```python
from build123d import *

# Parameters (mm, degrees)
SKETCH004_W     = 20
SKETCH004_H     = 8
PAD003_DEPTH    = 6
POCKET001_DEPTH = 5
SKETCH006_R     = 1.6
POCKET002_DEPTH = 11
FILLET004_R     = 3


with BuildPart() as part:
    # Sketch004 (on XY_Plane001 of Origin002) → Pad003 (new body)
    with BuildSketch(Plane.XY):
        Rectangle(SKETCH004_W, SKETCH004_H)
    extrude(amount=PAD003_DEPTH)

    # Sketch005 (on XZ_Plane001 of Origin002) → Pocket001 (cut, symmetric)
    with BuildSketch(Plane.XZ):
        with BuildLine():
            Line((-3.5, -2.936492), (3.5, -2.936492))
            ThreePointArc((3.5, -2.936492), (0, 3), (-3.5, -2.936492))
        make_face()
    extrude(amount=POCKET001_DEPTH, both=True, mode=Mode.SUBTRACT)

    # Sketch006 (on XY_Plane001 of Origin002) → Pocket002 (cut)
    with BuildSketch(Plane.XY):
        with Locations((-6.93, 0)):
            Circle(SKETCH006_R)
        with Locations((6.93, 0)):
            Circle(SKETCH006_R)
    extrude(amount=POCKET002_DEPTH, mode=Mode.SUBTRACT)

    # Fillet004
    fillet004_edges = [part.edges().sort_by_distance(p)[0] for p in [
        (10, 4, 3),
        (10, -4, 3),
        (-10, -4, 3),
        (-10, 4, 3),
    ]]
    fillet(fillet004_edges, radius=FILLET004_R)


solid = part.part
```
Build history of the part. All positions in model axes, mm. Give positions to 0.01 mm unless a question says otherwise; leave off trailing zeros. Loops run counter-clockwise (first coordinate to the right, second up) from the corner with the lowest first, then second, coordinate; pieces in that order, holes last. Notation, with made-up numbers: (-39.5, -24.5) -> (14.5, -24.5) arc R13 ccw to (14.5, -5.5) -> close; hole circle Ø1 at (20.25, -3.75). An arc over 180 degrees is marked (long way). One line per question, with ' | ' between items.
Q1. Cut at B-B, the plane y = 0. Write the cut outline in (x, z).
Filled sheet:
outline: (-10, 0) -> (-8.53, 0) -> (-8.53, 6) -> (-10, 6) -> close; (-5.33, 0) -> (-3.87, 0) arc R4 cw to (3.87, 0) -> (5.33, 0) -> (5.33, 6) -> (-5.33, 6) -> close; (8.53, 0) -> (10, 0) -> (10, 6) -> (8.53, 6) -> close
Q2. Cut at A-A, the plane z = 2.1. Write the cut outline in (x, y).
Filled sheet:
outline: (-10, -1) arc R3 ccw to (-7, -4) -> (-2.53, -4) -> (-2.53, 4) -> (-7, 4) arc R3 ccw to (-10, 1) -> close; (2.53, -4) -> (7, -4) arc R3 ccw to (10, -1) -> (10, 1) arc R3 ccw to (7, 4) -> (2.53, 4) -> close; hole circle Ø3.2 at (-6.93, 0); hole circle Ø3.2 at (6.93, 0)
Q3. Cut at D-D, the plane x = -6.5. Write the cut outline in (y, z), plus the area to 3 significant figures.
Filled sheet:
outline: (-4, 0) -> (-1.54, 0) -> (-1.54, 6) -> (-4, 6) -> close; (1.54, 0) -> (4, 0) -> (4, 6) -> (1.54, 6) -> close | area: 29.5 mm²
Q4. Drop flat-ended pins along their axis: pin 1 (1.5 mm diameter, centred on y = 3, z = 1, fed in from -X); pin 2 (1.9 mm diameter, centred on x = 6.93, y = 0, fed in from +Z); pin 3 (3 mm diameter, centred on x = 0, y = -1, fed in from -Z). Give the stop position or say it passes through.
Filled sheet:
pin 1: stops at x = -9.73 | pin 2: passes through | pin 3: stops at z = 2.71
Q5. Pull direction Y, two halves, no side cores. Call faces 1 (the flat face through (7, 2, 0)), 2 (the cylindrical face through (8.456, 0.481, 2.958)), 3 (the cylindrical face through (-9.14, -3.1, 3.04)), 4 (the cylindrical face through (-5.45, -0.61, 2.96)): pulls with the +Y half, pulls with the -Y half, needs draft (parallel to the pull), parting line crosses it, or undercut.
Filled sheet:
face 1: needs draft | face 2: undercut | face 3: pulls with the -Y half | face 4: undercut
Q6. Cut at C-C, the plane z = 5.5. Write the cut outline in (x, y), plus the area to 3 significant figures.
Filled sheet:
outline: (-10, -1) arc R3 ccw to (-7, -4) -> (7, -4) arc R3 ccw to (10, -1) -> (10, 1) arc R3 ccw to (7, 4) -> (-7, 4) arc R3 ccw to (-10, 1) -> close; hole circle Ø3.2 at (-6.93, 0); hole circle Ø3.2 at (6.93, 0) | area: 136 mm²
Q7. Drill centre lines: line 1 along X through (y, z) = (0, 4.35); line 2 along X through (y, z) = (0, 1.4); line 3 along Y through (x, z) = (-6.93, 2.9). Where is each one in solid material? Low to high. Write a range as [from, to].
Filled sheet:
line 1: x = [-10, -8.53], [-5.33, 5.33], [8.53, 10] | line 2: x = [-10, -8.53], [-5.33, -3.2], [3.2, 5.33], [8.53, 10] | line 3: y = [-4, -1.6], [1.6, 4]
